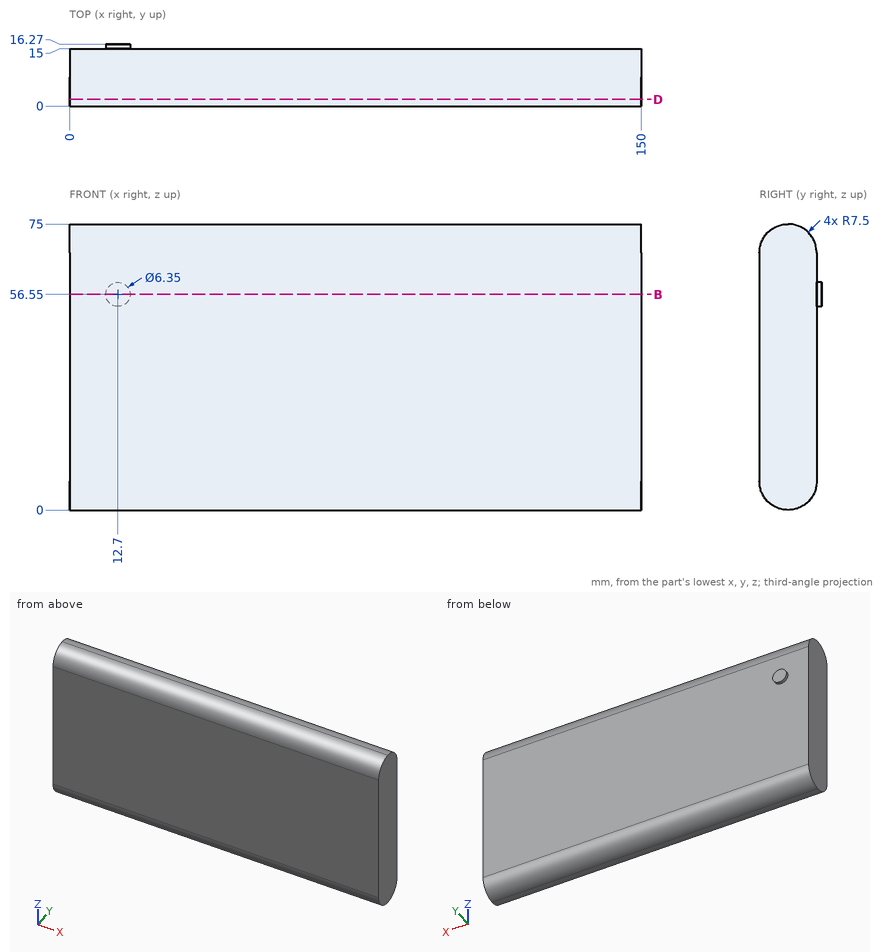
Study the drawing (mm; zero at the part's minimum x, y, z) and answer. Give positions to 0.01 mm unless a question says otherwise; leave off trailing zeros. Order: outer loops, then holes, each group sorted by start corner. A loop starts at its lowest first (then second) coordinate and runs counter-clockwise, first axis right, second up. Notation, with made-up numbers: M -20.75,43.25 L -15.75,43.25 A16 ccw -15.75,69.25 Z; hole C 16.5,-21 d11. An arc over 180 degrees is marked long. Put each result on its own line as item: value. Start each with the question number.
Item 1: Flat-ended cylindrical pins translate along their axes: P1, Ø8, axis at x = 111, z = 54, coming from the +Y side; P2, Ø4, axis at x = 27.5, y = 10.5, coming from the +Z side. Find the tip coordinate at first contact, or state that the pin passes through.
Item 2: The part is cut by section D-D, the plane y = 1.75. Determine the outline of the cut face in (x, z), and give its area (3 significant figures).
Item 3: The part is cut by section B-B, the plane z = 56.55. Determine the outline of the cut face in (x, y) (3 decimals), and give its area (3 significant figures).
Item 4: Find the intervals of material crossed by line 1 along Y through (x, z) = (25, 52); line 2 along X through (y, z) = (15.75, 54); line 3 along Z through (x, y) = (122.5, 5.25), in increasing order.
Answer key:
1. P1: stops at y = 15
1. P2: stops at z = 74.93
2. outline: M 0,2.68 L 150,2.68 L 150,72.32 L 0,72.32 Z
2. area: 10,400 mm²
3. outline: M 0,0 L 150,0 L 150,15 L 15.875,15 L 15.875,16.27 L 9.525,16.27 L 9.525,15 L 0,15 Z
3. area: 2,260 mm²
4. line 1: y = 0 to 15
4. line 2: x = 10.81 to 14.59
4. line 3: z = 0.35 to 74.65
